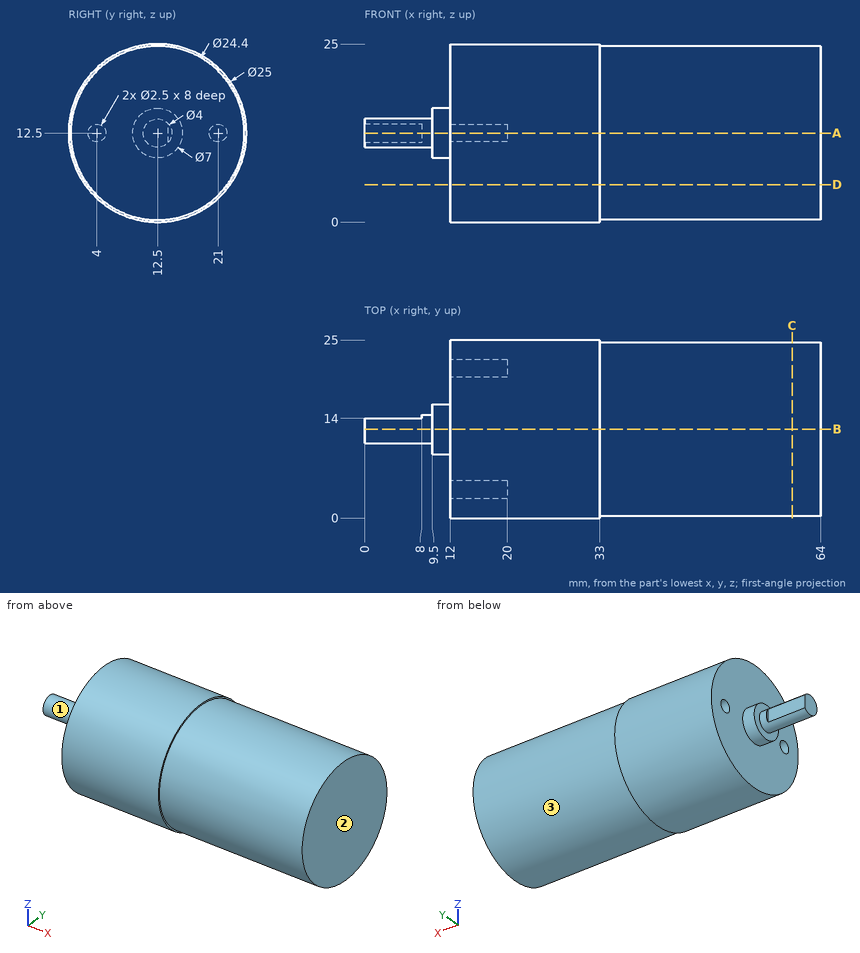
The figure shows three views and two pictorial views of one solid part (mm, origin at its lowest corner). Answer the questions. A direction names the side the tool comes from. Coordinates: 2 decimals unless noted, no trailing zeros. Loops run counter-clockwise (first coordinate to the right, second up) from the corner with the lowest first, then second, coordinate; pieces in that order, holes last.
1) Find section D-D on z = 5.25. Write down the section's boundary in (x, y).
2) Find the intervals of material crossed by L1, parallel to X at y = 21.5, z = 8.75; L2, parallel to Z at x = 27.5, y = 9.75; L3, parallel to Z at x = 31.5, y = 6.75, in increasing order.
3) A tool of negligible diameter and unlimited length cuts with its end or side. For the marked faces 1, 2 and 3, from which of +Z, -Z, +X, -X, +Y, -Y can it reach the whole face along a straight path? Write none if from no direction.
4) Find section A-A on z = 12.5. Write down the section's boundary in (x, y), then the cut area to 3 significant figures.
5) Flat-ended cylindrical pins translate along their axes: pin 1 Ø1.5 at (x, z) = (17, 22.5) entering from +Y; pin 2 Ø2 at (x, z) = (23, 7.5) entering from +Y; pin 3 Ø3 at (x, y) = (25, 6) entering from -Z. Find the tip coordinate at first contact, or state that the pin passes through.
6) Find section B-B on y = 12.5. Write down the section's boundary in (x, z).
7) Find section C-C on x = 60. Write down the section's boundary in (y, z).
Values:
1. outline: (12, 2.32) - (33, 2.32) - (33, 2.69) - (64, 2.69) - (64, 22.31) - (33, 22.31) - (33, 22.68) - (12, 22.68) - close
2. L1: x = 12 to 64
2. L2: z = 0.31 to 24.69
2. L3: z = 1.4 to 23.6
3. face 1: -X
3. face 2: +Z, -Z, +X, +Y, -Y
3. face 3: +X
4. outline: (0, 10.5) - (9.5, 10.5) - (9.5, 9) - (12, 9) - (12, 5.25) - (20, 5.25) - (20, 2.75) - (12, 2.75) - (12, 0) - (33, 0) - (33, 0.3) - (64, 0.3) - (64, 24.7) - (33, 24.7) - (33, 25) - (12, 25) - (12, 22.25) - (20, 22.25) - (20, 19.75) - (12, 19.75) - (12, 16) - (9.5, 16) - (9.5, 14.5) - (8, 14.5) - (8, 14) - (0, 14) - close
4. area: 1,290 mm2
5. pin 1: stops at y = 20.91
5. pin 2: stops at y = 24.34
5. pin 3: stops at z = 1.04
6. outline: (0, 10.5) - (9.5, 10.5) - (9.5, 9) - (12, 9) - (12, 0) - (33, 0) - (33, 0.3) - (64, 0.3) - (64, 24.7) - (33, 24.7) - (33, 25) - (12, 25) - (12, 16) - (9.5, 16) - (9.5, 14.5) - (0, 14.5) - close
7. outline: circle Ø24.4 at (12.5, 12.5)
